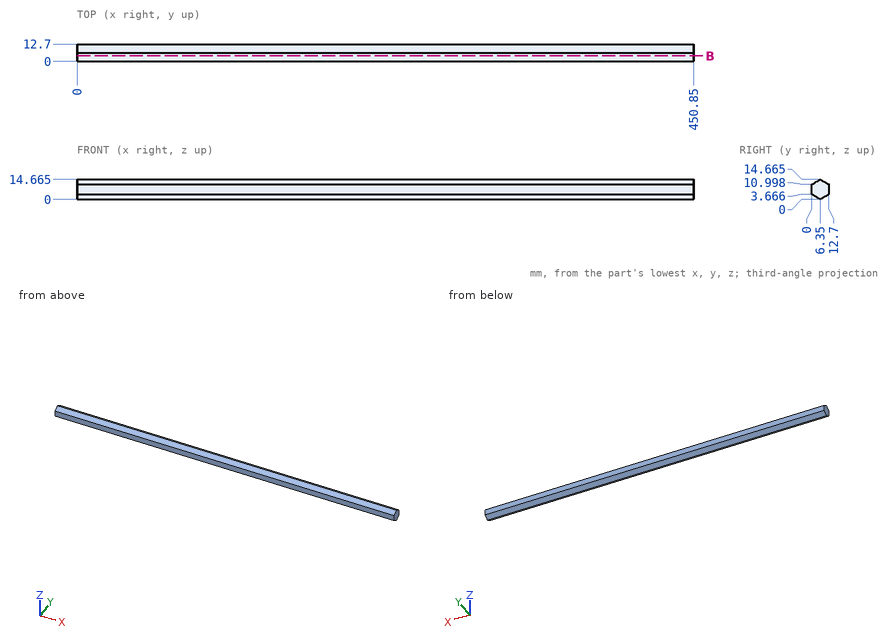
Job drawing, mm, ordinate dimensions from the low corner. One solid piece. Round coordinates to 2 decimals unless told otherwise and drop trailing zeros. Write each loop counter-clockwise with the first axis right and the second up, starting at its lowest first coordinate (ties: lowest second). Pieces come first, ordered by that corner, then holes. Notation, with made-up numbers: (79, -10) -> (118, -10) arc R34 ccw to (118, 20) -> close; hole circle Ø4 at (47.5, -8). An arc over 180 degrees is marked (long way). Answer as a JSON object with one key per item and string values.
(1) Band-saw the part on B-B, the plane y = 4. List the corners of the cut face in (x, z), then the cut area to 3 significant figures.
Reported:
{"outline": "(0, 1.36) -> (450.85, 1.36) -> (450.85, 13.31) -> (0, 13.31) -> close", "area": "5,390 mm^2"}
(2) Probe probe 1 along Z at (x, y) = (239, 6.25) (1 decimal); probe 2 along Y at (x, z) = (318.5, 11) (1 decimal); probe 3 along Z at (x, y) = (283.5, 4.5) (1 decimal). List the from-to ranges inside material, lowest first. Write a range as [from, to].
Reported:
{"probe 1": "z = [0.1, 14.6]", "probe 2": "y = [0, 12.7]", "probe 3": "z = [1.1, 13.6]"}
(3) Pin check, flat tips, straight feed: P1, Ø1, axis at x = 277, z = 3, coming from the +Y side (1 decimal); P2, Ø6, axis at x = 207, y = 9.5, coming from the +Z side; P3, Ø4, axis at x = 402, y = 11, coming from the +Z side (1 decimal). Stop position of each tip, or through.
Reported:
{"P1": "stops at y = 12.4", "P2": "stops at z = 14.58", "P3": "stops at z = 13.1"}
